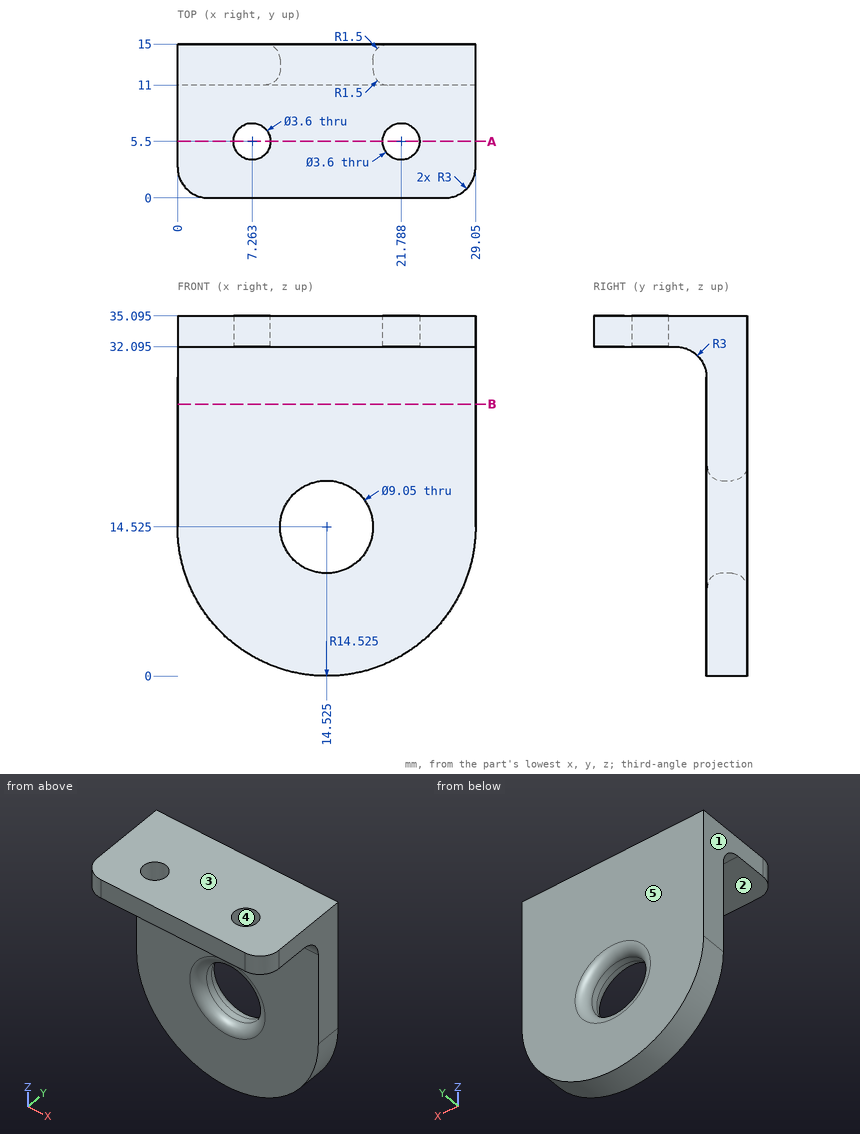
Study the drawing (mm; zero at the part's minimum x, y, z) and answer. A direction names the side the tool comes from. Give positions to 0.01 mm unless a question says otherwise; leave off trailing zeros. Order: outer loops, then holes, each group sorted by start corner. A loop starts at its lowest first (then second) coordinate and runs counter-clockwise, first axis right, second up. Notation, with made-up numbers: (14, -9.5) - (19, -9.5) arc R22 cw to (19, 16.5) - close; hole circle Ø9 at (-23, -16). An arc over 180 degrees is marked (long way). Answer as CSV lines item,"result". Start each with the question number.
Q1. For the marked faces 1 and 2, determine the directions among +Z, -Z, +X, -X, +Y, -Y from which every point of the face is accessible in a straight line to the end or side of a thin tool.
Q2. Given pin 1 Ø4.5 at (x, y) = (21.79, 5.5) entering from -Z (1 decimal); pin 2 Ø3 at (x, y) = (12, 11.5) entering from -Z; pin 3 Ø10.5 at (x, z) = (14.525, 14.525) entering from -Y (1 decimal), each flat-ended and moving along its own axis, determine where each tip first touches the part or whether it passes through.
Q3. The part is cut by section A-A (y = 5.5). Give the number of separate pieces and of enclosed holes in the cut face.
Q4. The mould has two halves that part along Y. Classify the marked faces 3, 4 and 5: +Y half, -Y half, draft (parallel to the pull), parting line (faces both ways), or undercut.
Q5. Find the intervals of material crossed by L1, parallel to Y at x = 9.5, z = 7; L2, parallel to Z at x = 3.5, y = 1 (1 decimal); L3, parallel to Z at x = 18, y = 13.75 (1 decimal), in increasing order. Write a range as [from, to].
Q6. The part is cut by section B-B (z = 26.5). Write down the section's boundary in (x, y), then the cut area to 3 significant figures.
Check result:
1,face 1,"+Z, -Z, -X, +Y, -Y"
1,face 2,"-Z, +X, -X, -Y"
2,pin 1,"stops at z = 32.1"
2,pin 2,"stops at z = 0.04"
2,pin 3,"stops at y = 11.2"
3,separate pieces,"3"
3,enclosed holes,"0"
4,face 3,"draft"
4,face 4,"undercut"
4,face 5,"+Y half"
5,L1,"y = [11, 15]"
5,L2,"z = [32.1, 35.1]"
5,L3,"z = [0.4, 11.6], [17.5, 35.1]"
6,outline,"(0, 11) - (29.05, 11) - (29.05, 15) - (0, 15) - close"
6,area,"116 mm²"
